Work out the finished part from the listing and answer in its coordinate system (mm). Face numbers are marked on the shaded views. Coordinates: 2 decimals unless noted, no trailing zeros. Write each loop counter-clockwise with the first axis right and the second up, starting at its lowest first coordinate (ties: lowest second). Pieces come first, ordered by that corner, then holes. Notation, with made-up numbers: (9, -0.75) -> (31, -0.75) arc R28 cw to (31, 29.25) -> close; hole circle Ø5 at (-20, -31). An arc over 180 degrees is marked (long way). Write each question's results on one line, items separated by ' | '. Start each with the question number.
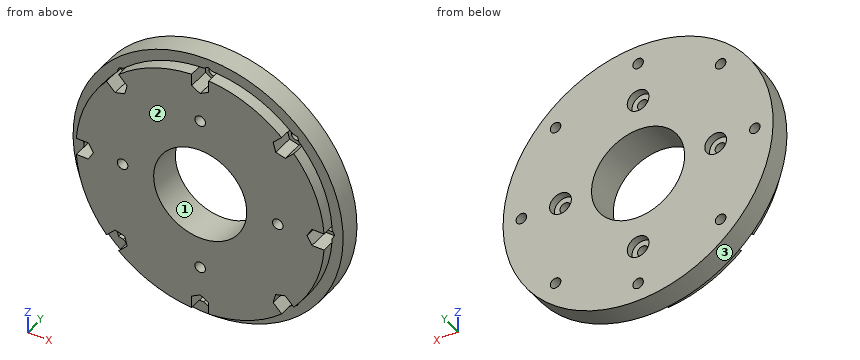
from build123d import *

# Parameters (mm, degrees)
CROQUIS1_R                                           = 40
CROQUIS1_R_2                                         = 15
SALIENTE_EXTRUIR1_DEPTH                              = 2
CROQUIS2_R                                           = 43.5
CROQUIS2_R_2                                         = 15
SALIENTE_EXTRUIR2_DEPTH                              = 7
TALADRO_DE_MARGEN_PARA_M31_D                         = 3.4
TALADRO_DE_MARGEN_PARA_M31_DEPTH                     = 20
TALADRO_DE_MARGEN_PARA_M31_TIP                       = 1.021463052
CORTAR_EXTRUIR1_START                                = -7
CORTAR_EXTRUIR1_DEPTH                                = 7
REFRENTADO_PARA_TORNILLO_CON_CABEZA_TRON_D           = 3.4
REFRENTADO_PARA_TORNILLO_CON_CABEZA_TRON_DEPTH       = 20
REFRENTADO_PARA_TORNILLO_CON_CABEZA_TRON_CBORE_D     = 7
REFRENTADO_PARA_TORNILLO_CON_CABEZA_TRON_CBORE_DEPTH = 2.4
REFRENTADO_PARA_TORNILLO_CON_CABEZA_TRON_TIP         = 1.021463052


with BuildPart() as part:
    # Croquis1 → Saliente-Extruir1 (new, symmetric)
    with BuildSketch(Plane(origin=(0, 0, 0), x_dir=(1, 0, 0), z_dir=(0, 1, 0))):
        with Locations(Location((0, 0, 0), (0, 0, 270))):
            Circle(CROQUIS1_R)
        with Locations(Location((0, 0, 0), (0, 0, 270))):
            Circle(CROQUIS1_R_2, mode=Mode.SUBTRACT)
    extrude(amount=SALIENTE_EXTRUIR1_DEPTH, both=True)

    # Croquis2 → Saliente-Extruir2 (add)
    with BuildSketch(Plane(origin=(0, 2, 0), x_dir=(1, 0, 0), z_dir=(0, 1, 0))):
        with Locations(Location((0, 0, 0), (0, 0, 270))):
            Circle(CROQUIS2_R)
        with Locations(Location((0, 0, 0), (0, 0, 270))):
            Circle(CROQUIS2_R_2, mode=Mode.SUBTRACT)
    extrude(amount=SALIENTE_EXTRUIR2_DEPTH)

    # Taladro de margen para M31
    with Locations(Plane(origin=(0, 9, 0), x_dir=(1, 0, 0), z_dir=(0, 1, 0))):
        with Locations((0, 37.6), (26.587214973, 26.587214973), (37.6, 0), (26.587214973, -26.587214973), (0, -37.6), (-26.587214973, -26.587214973), (-37.6, 0), (-26.587214973, 26.587214973)):
            Hole(TALADRO_DE_MARGEN_PARA_M31_D / 2, depth=TALADRO_DE_MARGEN_PARA_M31_DEPTH)
            with Locations((0, 0, -(TALADRO_DE_MARGEN_PARA_M31_DEPTH + TALADRO_DE_MARGEN_PARA_M31_TIP / 2))):  # 118° drill point
                Cone(0, TALADRO_DE_MARGEN_PARA_M31_D / 2, TALADRO_DE_MARGEN_PARA_M31_TIP, mode=Mode.SUBTRACT)

    # Croquis5 → Cortar-Extruir1 (cut)
    with BuildSketch(Plane.XZ.offset(2).offset(CORTAR_EXTRUIR1_START)):
        with BuildLine():
            Line((-2.753960784, 39.19), (-2.753960784, 36.01))
            Line((-2.753960784, 36.01), (0, 34.42))
            Line((0, 34.42), (2.753960784, 36.01))
            Line((2.753960784, 36.01), (2.753960784, 39.19))
            Line((2.753960784, 39.19), (2.753960784, 39.905083636))
            ThreePointArc((2.753960784, 39.905083636), (2.073794244, 39.946206046), (1.393025891, 39.975736127))
            Line((1.393025891, 39.975736127), (0, 40.78))
            Line((0, 40.78), (-1.393025891, 39.975736127))
            ThreePointArc((-1.393025891, 39.975736127), (-2.073794244, 39.946206046), (-2.753960784, 39.905083636))
            Line((-2.753960784, 39.905083636), (-2.753960784, 39.19))
        make_face()
        with BuildLine():
            Line((25.764170409, 29.6588591), (23.515570845, 27.410259536))
            Line((23.515570845, 27.410259536), (24.338615408, 24.338615408))
            Line((24.338615408, 24.338615408), (27.410259536, 23.515570845))
            Line((27.410259536, 23.515570845), (29.6588591, 25.764170409))
            Line((29.6588591, 25.764170409), (30.164499588, 26.269810897))
            ThreePointArc((30.164499588, 26.269810897), (29.71262715, 26.779839205), (29.252132152, 27.282096044))
            Line((29.252132152, 27.282096044), (28.835814537, 28.835814537))
            Line((28.835814537, 28.835814537), (27.282096044, 29.252132152))
            ThreePointArc((27.282096044, 29.252132152), (26.779839205, 29.71262715), (26.269810897, 30.164499588))
            Line((26.269810897, 30.164499588), (25.764170409, 29.6588591))
        make_face()
        with BuildLine():
            Line((39.19, 2.753960784), (36.01, 2.753960784))
            Line((36.01, 2.753960784), (34.42, 0))
            Line((34.42, 0), (36.01, -2.753960784))
            Line((36.01, -2.753960784), (39.19, -2.753960784))
            Line((39.19, -2.753960784), (39.905083636, -2.753960784))
            ThreePointArc((39.905083636, -2.753960784), (39.946206046, -2.073794244), (39.975736127, -1.393025891))
            Line((39.975736127, -1.393025891), (40.78, 0))
            Line((40.78, 0), (39.975736127, 1.393025891))
            ThreePointArc((39.975736127, 1.393025891), (39.946206046, 2.073794244), (39.905083636, 2.753960784))
            Line((39.905083636, 2.753960784), (39.19, 2.753960784))
        make_face()
        with BuildLine():
            Line((29.6588591, -25.764170409), (27.410259536, -23.515570845))
            Line((27.410259536, -23.515570845), (24.338615408, -24.338615408))
            Line((24.338615408, -24.338615408), (23.515570845, -27.410259536))
            Line((23.515570845, -27.410259536), (25.764170409, -29.6588591))
            Line((25.764170409, -29.6588591), (26.269810897, -30.164499588))
            ThreePointArc((26.269810897, -30.164499588), (26.779839205, -29.71262715), (27.282096044, -29.252132152))
            Line((27.282096044, -29.252132152), (28.835814537, -28.835814537))
            Line((28.835814537, -28.835814537), (29.252132152, -27.282096044))
            ThreePointArc((29.252132152, -27.282096044), (29.71262715, -26.779839205), (30.164499588, -26.269810897))
            Line((30.164499588, -26.269810897), (29.6588591, -25.764170409))
        make_face()
        with BuildLine():
            Line((2.753960784, -39.19), (2.753960784, -36.01))
            Line((2.753960784, -36.01), (0, -34.42))
            Line((0, -34.42), (-2.753960784, -36.01))
            Line((-2.753960784, -36.01), (-2.753960784, -39.19))
            Line((-2.753960784, -39.19), (-2.753960784, -39.905083636))
            ThreePointArc((-2.753960784, -39.905083636), (-2.073794244, -39.946206046), (-1.393025891, -39.975736127))
            Line((-1.393025891, -39.975736127), (0, -40.78))
            Line((0, -40.78), (1.393025891, -39.975736127))
            ThreePointArc((1.393025891, -39.975736127), (2.073794244, -39.946206046), (2.753960784, -39.905083636))
            Line((2.753960784, -39.905083636), (2.753960784, -39.19))
        make_face()
        with BuildLine():
            Line((-25.764170409, -29.6588591), (-23.515570845, -27.410259536))
            Line((-23.515570845, -27.410259536), (-24.338615408, -24.338615408))
            Line((-24.338615408, -24.338615408), (-27.410259536, -23.515570845))
            Line((-27.410259536, -23.515570845), (-29.6588591, -25.764170409))
            Line((-29.6588591, -25.764170409), (-30.164499588, -26.269810897))
            ThreePointArc((-30.164499588, -26.269810897), (-29.71262715, -26.779839205), (-29.252132152, -27.282096044))
            Line((-29.252132152, -27.282096044), (-28.835814537, -28.835814537))
            Line((-28.835814537, -28.835814537), (-27.282096044, -29.252132152))
            ThreePointArc((-27.282096044, -29.252132152), (-26.779839205, -29.71262715), (-26.269810897, -30.164499588))
            Line((-26.269810897, -30.164499588), (-25.764170409, -29.6588591))
        make_face()
        with BuildLine():
            Line((-39.19, -2.753960784), (-36.01, -2.753960784))
            Line((-36.01, -2.753960784), (-34.42, 0))
            Line((-34.42, 0), (-36.01, 2.753960784))
            Line((-36.01, 2.753960784), (-39.19, 2.753960784))
            Line((-39.19, 2.753960784), (-39.905083636, 2.753960784))
            ThreePointArc((-39.905083636, 2.753960784), (-39.946206046, 2.073794244), (-39.975736127, 1.393025891))
            Line((-39.975736127, 1.393025891), (-40.78, 0))
            Line((-40.78, 0), (-39.975736127, -1.393025891))
            ThreePointArc((-39.975736127, -1.393025891), (-39.946206046, -2.073794244), (-39.905083636, -2.753960784))
            Line((-39.905083636, -2.753960784), (-39.19, -2.753960784))
        make_face()
        with BuildLine():
            Line((-29.6588591, 25.764170409), (-27.410259536, 23.515570845))
            Line((-27.410259536, 23.515570845), (-24.338615408, 24.338615408))
            Line((-24.338615408, 24.338615408), (-23.515570845, 27.410259536))
            Line((-23.515570845, 27.410259536), (-25.764170409, 29.6588591))
            Line((-25.764170409, 29.6588591), (-26.269810897, 30.164499588))
            ThreePointArc((-26.269810897, 30.164499588), (-26.779839205, 29.71262715), (-27.282096044, 29.252132152))
            Line((-27.282096044, 29.252132152), (-28.835814537, 28.835814537))
            Line((-28.835814537, 28.835814537), (-29.252132152, 27.282096044))
            ThreePointArc((-29.252132152, 27.282096044), (-29.71262715, 26.779839205), (-30.164499588, 26.269810897))
            Line((-30.164499588, 26.269810897), (-29.6588591, 25.764170409))
        make_face()
    extrude(amount=CORTAR_EXTRUIR1_DEPTH, mode=Mode.SUBTRACT)

    # Refrentado para tornillo con cabeza troncocónica de M32
    with Locations(Plane(origin=(0, 9, 0), x_dir=(1, 0, 0), z_dir=(0, 1, 0))):
        with Locations((0, 25), (25, 0), (0, -25), (-25, 0)):
            CounterBoreHole(REFRENTADO_PARA_TORNILLO_CON_CABEZA_TRON_D / 2, REFRENTADO_PARA_TORNILLO_CON_CABEZA_TRON_CBORE_D / 2, REFRENTADO_PARA_TORNILLO_CON_CABEZA_TRON_CBORE_DEPTH, depth=REFRENTADO_PARA_TORNILLO_CON_CABEZA_TRON_DEPTH)
            with Locations((0, 0, -(REFRENTADO_PARA_TORNILLO_CON_CABEZA_TRON_DEPTH + REFRENTADO_PARA_TORNILLO_CON_CABEZA_TRON_TIP / 2))):  # 118° drill point
                Cone(0, REFRENTADO_PARA_TORNILLO_CON_CABEZA_TRON_D / 2, REFRENTADO_PARA_TORNILLO_CON_CABEZA_TRON_TIP, mode=Mode.SUBTRACT)


solid = part.part
1. Find section D-D on x = -8.5. Give the vertices of the cut face in (y, z), and give its area (3 significant figures).
2. Find section A-A on z = 37.6. Give the vertices of the cut face in (x, y), and give its area (3 significant figures).
3. Find section B-B on x = 37.6. Give the vertices of the cut face in (y, z).
4. Determine the mould class of the marked faces 1, 2 and 3 for opening direction Z: pulls with the +Z half, pulls with the -Z half, needs draft (parallel to the pull), parting line crosses it, or undercut.
5. Given pin 1 Ø2 at (x, z) = (25, 0) entering from +Y; pin 2 Ø3 at (x, y) = (-5.5, 3.5) entering from -Z; pin 3 Ø6 at (x, y) = (-16, 3) entering from +Z; pin 4 Ø1.7 at (x, z) = (0, -36.5) entering from -Y, each flat-ended and moving along its own axis, determine where each tip first touches the part or whether it passes through.
6. Find section C-C on y = 0.5. Give the number of separate pieces and of enclosed holes in the cut face, and give its area (3 significant figures).
7. Find the intervals of material crossed by L1, parallel to Z at x = 25, y = 0.5; L2, parallel to Z at x = 1.5, y = 8; L3, parallel to Y at x = 37, z = 19.5, in increasing order.
Ans:
1) outline: (-2, -39.09) -> (2, -39.09) -> (2, -42.66) -> (9, -42.66) -> (9, -12.36) -> (-2, -12.36) -> close; (-2, 12.36) -> (9, 12.36) -> (9, 42.66) -> (2, 42.66) -> (2, 39.09) -> (-2, 39.09) -> close | area: 638 mm²
2) outline: (-21.87, 2) -> (-13.65, 2) -> (-13.65, -2) -> (-2.75, -2) -> (-2.75, 5) -> (-1.7, 5) -> (-1.7, 9) -> (-21.87, 9) -> close; (1.7, 5) -> (2.75, 5) -> (2.75, -2) -> (13.65, -2) -> (13.65, 2) -> (21.87, 2) -> (21.87, 9) -> (1.7, 9) -> close | area: 363 mm²
3) outline: (-2, -13.65) -> (2, -13.65) -> (2, -21.87) -> (9, -21.87) -> (9, -1.7) -> (5, -1.7) -> (5, -2.75) -> (-2, -2.75) -> close; (-2, 2.75) -> (5, 2.75) -> (5, 1.7) -> (9, 1.7) -> (9, 21.87) -> (2, 21.87) -> (2, 13.65) -> (-2, 13.65) -> close
4) face 1: undercut | face 2: needs draft | face 3: parting line crosses it
5) pin 1: passes through | pin 2: stops at z = -43.32 | pin 3: stops at z = 41.51 | pin 4: stops at y = 5
6) separate pieces: 1 | enclosed holes: 5 | area: 4,070 mm²
7) L1: z = -31.22 to -28.89, -24.16 to -1.7, 1.7 to 24.16, 28.89 to 31.22 | L2: z = -43.47 to -38.4, -36.8 to -28.16, -21.84 to -14.92, 14.92 to 21.84, 28.16 to 36.8, 38.4 to 43.47 | L3: y = 2 to 9
